Input: part model. Units: mm. Frame: model coordinates. A direction names the side the tool comes from. Coordinates: 2 decimals unless noted, no trailing zeros. Loops run counter-clockwise (first coordinate to the right, second up) from the corner with the lowest first, then second, coordinate; pieces in that order, holes last.
Autodesk Fusion 360 part; units mm, degrees
sketch "Sketch1" plane through (0, 0, 0) normal (0, 0, 1) x (1, 0, 0) in component "PJ3F07-5P"
  circle A0 centre (0, 0) radius 1.8
  circle A1 centre (0, 0) radius 3
  dimension "d1" = 3.6
  dimension "d2" = 6
extrude "Extrude1" add sketch "Sketch1" against normal blind 3 in component "PJ3F07-5P"
ref_plane "WorkPlane1" through (0, 0, -2) normal (0, 0, -1) x (-1, 0, 0) in component "PJ3F07-5P"
sketch "Sketch2" plane through (0, 0, -2) normal (0, 0, -1) x (-1, 0, 0) in component "PJ3F07-5P"
  line L0 (-4.5, 2.5) -> (4.5, 2.5)
  line L1 (4.5, 2.5) -> (4.5, -2.5)
  line L2 (4.5, -2.5) -> (-4.5, -2.5)
  line L3 (-4.5, -2.5) -> (-4.5, 2.5)
  line L4 (-4.5, 2.5) -> (4.5, -2.5) construction
  line L5 (4.5, 2.5) -> (-4.5, -2.5) construction
  circle A0 centre (0, 0) radius 1.8
  circle A1 centre (0, 0) radius 3
  dimension "d6" = 9
  dimension "d7" = 5
extrude "Extrude2" add sketch "Sketch2" along normal blind 1 contours L0 L2 L3 A1 | L0 L1 L2 A1 in component "PJ3F07-5P"
sketch "Sketch3" plane through (0, 0, -3) normal (0, 0, -1) x (-1, 0, 0) in component "PJ3F07-5P"
  circle A0 centre (0, 0) radius 1.8
  arc A1 (-1.6583, -2.5) -> (1.6583, -2.5) centre (0, 0) ccw
  line L0 (1.6583, -2.5) -> (4.5, -2.5)
  line L1 (4.5, -2.5) -> (4.5, 2.5)
  line L2 (4.5, 2.5) -> (1.6583, 2.5)
  arc A2 (1.6583, 2.5) -> (-1.6583, 2.5) centre (0, 0) ccw
  line L3 (-1.6583, 2.5) -> (-4.5, 2.5)
  line L4 (-4.5, 2.5) -> (-4.5, -2.5)
  line L5 (-4.5, -2.5) -> (-1.6583, -2.5)
  line L6 (6, 2.5) -> (-6, 2.5)
  line L7 (-6, 2.5) -> (-6, -2.5)
  line L8 (-6, -2.5) -> (6, -2.5)
  line L9 (6, -2.5) -> (6, 2.5)
  line L10 (6, 2.5) -> (-6, -2.5) construction
  line L11 (-6, 2.5) -> (6, -2.5) construction
  dimension "d10" = 12
  dimension "d11" = 5
extrude "Extrude3" add sketch "Sketch3" along normal blind 11 contours L0 L1 L2 L3 L4 L5 L6 L8 | L4 L6 L7 L8 | L1 L6 L8 L9 in component "PJ3F07-5P"
sketch "Sketch4" plane through (0, -2.5, 0) normal (0, -1, 0) x (1, 0, 0) in component "PJ3F07-5P"
  line L0 (-1.6583, -2) -> (-4.5, -2)
  line L1 (-4.5, -2) -> (-4.5, -3)
  line L2 (-4.5, -3) -> (-6, -3)
  line L3 (-6, -3) -> (-6, -14)
  line L4 (-6, -14) -> (6, -14)
  line L5 (6, -14) -> (6, -3)
  line L6 (6, -3) -> (4.5, -3)
  line L7 (4.5, -3) -> (4.5, -2)
  line L8 (4.5, -2) -> (1.6583, -2)
  line L9 (1.6583, -2) -> (1.6583, -3)
  line L10 (1.6583, -3) -> (-1.6583, -3)
  line L11 (-1.6583, -3) -> (-1.6583, -2)
  circle A0 centre (5, -4) radius 0.5
  circle A1 centre (5, -6.5) radius 0.5
  circle A2 centre (-5, -4) radius 0.5
  circle A3 centre (-5, -6.5) radius 0.5
  circle A4 centre (0, -11.5) radius 0.5
  line L12 (0.75, -6.9) -> (-0.75, -6.9)
  line L13 (-0.75, -6.9) -> (-0.75, -6.1)
  line L14 (-0.75, -6.1) -> (0.75, -6.1)
  line L15 (0.75, -6.1) -> (0.75, -6.9)
  line L16 (0.75, -6.9) -> (-0.75, -6.1) construction
  line L17 (-0.75, -6.9) -> (0.75, -6.1) construction
  line L18 (-2.9, -12.25) -> (-2.1, -12.25)
  line L19 (-2.1, -12.25) -> (-2.1, -10.75)
  line L20 (-2.1, -10.75) -> (-2.9, -10.75)
  line L21 (-2.9, -10.75) -> (-2.9, -12.25)
  line L22 (-2.9, -12.25) -> (-2.1, -10.75) construction
  line L23 (-2.1, -12.25) -> (-2.9, -10.75) construction
  line L24 (-5.4, -12.25) -> (-4.6, -12.25)
  line L25 (-4.6, -12.25) -> (-4.6, -10.75)
  line L26 (-4.6, -10.75) -> (-5.4, -10.75)
  line L27 (-5.4, -10.75) -> (-5.4, -12.25)
  line L28 (-5.4, -12.25) -> (-4.6, -10.75) construction
  line L29 (-4.6, -12.25) -> (-5.4, -10.75) construction
  line L30 (4.6, -12.25) -> (5.4, -12.25)
  line L31 (5.4, -12.25) -> (5.4, -10.75)
  line L32 (5.4, -10.75) -> (4.6, -10.75)
  line L33 (4.6, -10.75) -> (4.6, -12.25)
  line L34 (4.6, -12.25) -> (5.4, -10.75) construction
  line L35 (5.4, -12.25) -> (4.6, -10.75) construction
  line L36 (2.1, -12.25) -> (2.9, -12.25)
  line L37 (2.9, -12.25) -> (2.9, -10.75)
  line L38 (2.9, -10.75) -> (2.1, -10.75)
  line L39 (2.1, -10.75) -> (2.1, -12.25)
  line L40 (2.1, -12.25) -> (2.9, -10.75) construction
  line L41 (2.9, -12.25) -> (2.1, -10.75) construction
  line L42 (-1.6583, -2) -> (1.6583, -2) construction
  line L43 (0, -2) -> (0, -14) construction
  line L44 (-5, -14) -> (-5, -3) construction
  line L45 (5, -14) -> (5, -3) construction
  line L46 (5.1, -11) -> (4.9, -11)
  line L47 (4.9, -11) -> (4.9, -12)
  line L48 (4.9, -12) -> (5.1, -12)
  line L49 (5.1, -12) -> (5.1, -11)
  line L50 (5.1, -11) -> (4.9, -12) construction
  line L51 (4.9, -11) -> (5.1, -12) construction
  line L52 (2.6, -11) -> (2.4, -11)
  line L53 (2.4, -11) -> (2.4, -12)
  line L54 (2.4, -12) -> (2.6, -12)
  line L55 (2.6, -12) -> (2.6, -11)
  line L56 (2.6, -11) -> (2.4, -12) construction
  line L57 (2.4, -11) -> (2.6, -12) construction
  line L58 (-2.4, -11) -> (-2.6, -11)
  line L59 (-2.6, -11) -> (-2.6, -12)
  line L60 (-2.6, -12) -> (-2.4, -12)
  line L61 (-2.4, -12) -> (-2.4, -11)
  line L62 (-2.4, -11) -> (-2.6, -12) construction
  line L63 (-2.6, -11) -> (-2.4, -12) construction
  line L64 (-4.9, -11) -> (-5.1, -11)
  line L65 (-5.1, -11) -> (-5.1, -12)
  line L66 (-5.1, -12) -> (-4.9, -12)
  line L67 (-4.9, -12) -> (-4.9, -11)
  line L68 (-4.9, -11) -> (-5.1, -12) construction
  line L69 (-5.1, -11) -> (-4.9, -12) construction
  line L70 (0.5, -6.4) -> (-0.5, -6.4)
  line L71 (-0.5, -6.4) -> (-0.5, -6.6)
  line L72 (-0.5, -6.6) -> (0.5, -6.6)
  line L73 (0.5, -6.6) -> (0.5, -6.4)
  line L74 (0.5, -6.4) -> (-0.5, -6.6) construction
  line L75 (-0.5, -6.4) -> (0.5, -6.6) construction
  circle A5 centre (-5, -4) radius 0.4
  circle A6 centre (-5, -6.5) radius 0.4
  circle A7 centre (0, -11.5) radius 0.4
  circle A8 centre (5, -6.5) radius 0.4
  circle A9 centre (5, -4) radius 0.4
  point P0 (0, -6.5)
  point P1 (-2.5, -11.5)
  point P2 (-5, -11.5)
  point P3 (5, -11.5)
  point P4 (2.5, -11.5)
  point P5 (5, -11.5)
  point P6 (2.5, -11.5)
  point P7 (-2.5, -11.5)
  point P8 (-5, -11.5)
  point P9 (0, -6.5)
  dimension "d14" = 1
  dimension "d15" = 1
  dimension "d16" = 1
  dimension "d17" = 1
  dimension "d18" = 1
  dimension "d19" = 1
  dimension "d20" = 0.8
  dimension "d21" = 1.5
  dimension "d23" = 2.5
  dimension "d24" = 4.5
  dimension "d25" = 1
  dimension "d26" = 2.5
  dimension "d27" = 1.5
  dimension "d28" = 0.8
  dimension "d29" = 0.8
  dimension "d30" = 1.5
  dimension "d31" = 1.5
  dimension "d32" = 0.8
  dimension "d33" = 0.8
  dimension "d34" = 1.5
  dimension "d35" = 5
  dimension "d36" = 2.5
  dimension "d37" = 10
  dimension "d38" = 5
  dimension "d39" = 5
  dimension "d40" = 9.5
  dimension "d41" = 9.5
  dimension "d42" = 9.5
  dimension "d43" = 9.5
  dimension "d44" = 1
  dimension "d45" = 1
  dimension "d48" = 0.2
  dimension "d49" = 1
  dimension "d50" = 1
  dimension "d51" = 0.2
  dimension "d52" = 0.2
  dimension "d53" = 1
  dimension "d54" = 0.2
  dimension "d55" = 1
  dimension "d56" = 1
  dimension "d57" = 0.2
  dimension "d58" = 0.8
  dimension "d59" = 0.8
  dimension "d60" = 0.8
  dimension "d61" = 0.8
  dimension "d62" = 0.8
extrude "Extrude5" add sketch "Sketch4" along normal blind 1 contours A5 | A6 | A7 | A8 | A9 in component "PJ3F07-5P"
extrude "Extrude6" add sketch "Sketch4" along normal blind 3.5 contours L46 L47 L48 L49 | L52 L53 L54 L55 | L58 L59 L60 L61 | L64 L65 L66 L67 | L70 L71 L72 L73 in component "PJ3F07-5P"
fillet "Fillet1" radius 0.5 10 edges at (-5, -6, -12) (-5, -6, -11) (-2.5, -6, -12) (-2.5, -6, -11) (2.5, -6, -12) (2.5, -6, -11) (5, -6, -12) (5, -6, -11) (0.5, -6, -6.5) (-0.5, -6, -6.5) in component "PJ3F07-5P"
component "PJ3F07-5P" placed x (1, 0, 0) y (0, 1, 0) z (0, 0, 1) at (0, 0, 0)
Item 1: Section query C-C (y = 0). Output: boundary loops of the cut face in (x, z), then the cut area to 3 significant figures.
Result:
outline: (-6, -14) - (-1.8, -14) - (-1.8, 0) - (-3, 0) - (-3, -2) - (-4.5, -2) - (-4.5, -3) - (-6, -3) - close; (1.8, -14) - (6, -14) - (6, -3) - (4.5, -3) - (4.5, -2) - (3, -2) - (3, 0) - (1.8, 0) - close
area: 103 mm2
Item 2: Line query: L1, parallel to X at y = 0, z = -6.75; L2, parallel to Y at x = 0, z = -8.75; L3, parallel to Y at x = 0, z = -1.1. Output: solid intervals per line, ascending.
Result:
L1: x = -6 to -1.8, 1.8 to 6
L2: y = -2.5 to -1.8, 1.8 to 2.5
L3: y = -3 to -1.8, 1.8 to 3
Item 3: Section query B-B (z = -4). Output: boundary loops of the cut face in (x, y), then the cut area to 3 significant figures.
Result:
outline: (-6, -2.5) - (-5.4, -2.5) - (-5.4, -3.5) - (-4.6, -3.5) - (-4.6, -2.5) - (4.6, -2.5) - (4.6, -3.5) - (5.4, -3.5) - (5.4, -2.5) - (6, -2.5) - (6, 2.5) - (-6, 2.5) - close; hole circle Ø3.6 at (0, 0)
area: 51.4 mm2
Item 4: Section query D-D (x = -0.75). Output: boundary loops of the cut face in (y, z).
Result:
outline: (-2.9, -3) - (-2.5, -3) - (-2.5, -14) - (-1.64, -14) - (-1.64, 0) - (-2.9, 0) - close; (1.64, -14) - (2.5, -14) - (2.5, -3) - (2.9, -3) - (2.9, 0) - (1.64, 0) - close
Item 5: Reachability of faces 4 (the face through (5, -3.5, -4)), 5 (the face through (2.6, -4.2, -11.5)), 6 (the face through (0, -4, -6.6)), 7 (the face through (5.1, -4.2, -11.5)) from +Z, -Z, +X, -X, +Y, -Y: full face, straight path, thin tool, end or side. Return the list, or none.
Result:
face 4: +Z, +X, -X, -Y
face 5: +Z, -Z, -Y
face 6: -Y
face 7: -Z, +X, -Y
Item 6: Section query A-A (y = -3.75). Output: boundary loops of the cut face in (x, z), then the cut area to 4 significant figures.
Result:
outline: (-5.1, -12) - (-4.9, -12) - (-4.9, -11) - (-5.1, -11) - close; (-2.6, -12) - (-2.4, -12) - (-2.4, -11) - (-2.6, -11) - close; (-0.5, -6.6) - (0.5, -6.6) - (0.5, -6.4) - (-0.5, -6.4) - close; (2.4, -12) - (2.6, -12) - (2.6, -11) - (2.4, -11) - close; (4.9, -12) - (5.1, -12) - (5.1, -11) - (4.9, -11) - close
area: 1.000 mm2
Item 7: Mould query, pull axis X, two halves, no side actions, for faces 1 (the face through (-5.052, -2.993, -6.897)), 2 (the face through (-6, 0, -8)), 3 (the face through (5, -3.5, -6.5)). Classes: +X half, -X half, draft (parallel to the pull), parting line (faces both ways), or undercut.
Result:
face 1: undercut
face 2: -X half
face 3: draft
Item 8: Contact query for flat-ended pins moving along their axis: P1, Ø0.5, axis at y = -1, z = -2.5, coming from the -X side; P2, Ø3, axis at x = 3, z = -5.5, coming from the -Y side; P3, Ø1.6, axis at x = 5.5, y = 0, coming from the +Z side. Output: stop coordinate, or through.
Result:
P1: stops at x = -4.5
P2: stops at y = -2.5
P3: stops at z = -3
